The drawing under review shows one solid part. Ordinate dimensions are in mm from its lowest x, y, z. A direction names the side the tool comes from. Coordinates: 2 decimals unless noted, no trailing zeros. Order: outer loops, then holes, each group sorted by start corner. A loop starts at its lowest first (then second) coordinate and runs counter-clockwise, first axis right, second up.
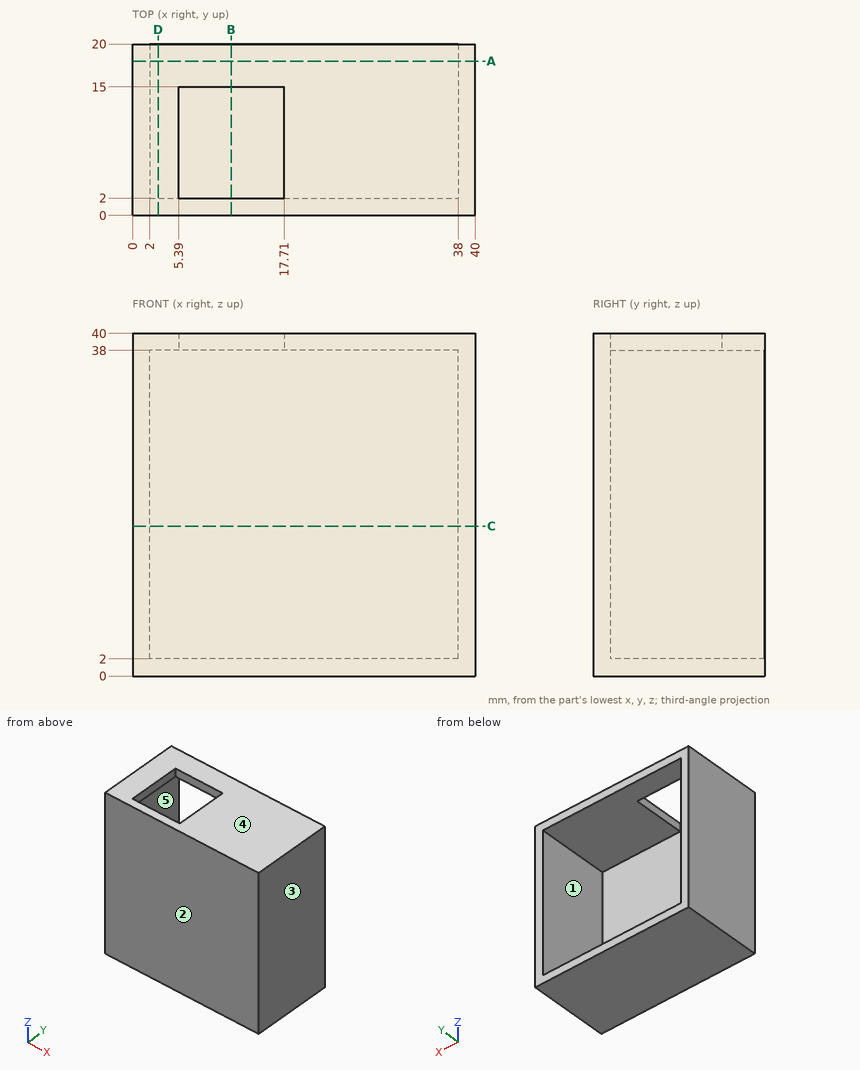
1. Add section C-C (z = 17.5). Give the boundary of the cut face in (x, y).
2. Add section A-A (y = 18). Give the boundary of the cut face in (x, z).
3. Insertion check: pin 1 (6 mm diameter, centred on x = 10, z = 22, fed in from +Y). The pin has a flat end and moves straight along its axis. Give the tip position at first contact, or say it passes through.
4. For the marked faces 1 and 2, list the 3-axis set-ups (+Z, -Z, +X, -X, +Y, -Y) from which the entire face can be reached by the end or side of a thin tool; tool diameter is ignored.
5. Mouldability with a two-part tool opening along Z and no side actions: class the marked faces 3, 4 and 5 as pulls with the +Z half, pulls with the -Z half, needs draft (parallel to the pull), parting line crosses it, or undercut.
6. Add section D-D (x = 3). Give the boundary of the cut face in (y, z).
7. Add section B-B (x = 11.5). Give the boundary of the cut face in (y, z), and give its area (3 significant figures).
8. To check wall thickness, follow line 1 (Z direction, x = 5, y = 6.75); line 2 (Y direction, x = 21, z = 34). State the ranges of each line that lie inside material, in increasing order.
Solution:
1. outline: (0, 0) - (40, 0) - (40, 20) - (38, 20) - (38, 2) - (2, 2) - (2, 20) - (0, 20) - close
2. outline: (0, 0) - (40, 0) - (40, 40) - (0, 40) - close; hole (2, 2) - (38, 2) - (38, 38) - (2, 38) - close
3. pin 1: stops at y = 2
4. face 1: +Y
4. face 2: +Z, -Z, +X, -X, -Y
5. face 3: needs draft
5. face 4: pulls with the +Z half
5. face 5: undercut
6. outline: (0, 0) - (20, 0) - (20, 2) - (2, 2) - (2, 38) - (20, 38) - (20, 40) - (0, 40) - close
7. outline: (0, 0) - (20, 0) - (20, 2) - (2, 2) - (2, 40) - (0, 40) - close; (15, 38) - (20, 38) - (20, 40) - (15, 40) - close
7. area: 126 mm2
8. line 1: z = 0 to 2, 38 to 40
8. line 2: y = 0 to 2
